from build123d import *

# Parameters (mm, degrees)
BOSS_EXTRUDE1_DEPTH       = 3.175
F_6_CLEARANCE_HOLE1_D     = 3.7973
F_6_CLEARANCE_HOLE1_DEPTH = 6.35
F_6_CLEARANCE_HOLE1_TIP   = 1.140824014
FILLET1_R                 = 1.27


with BuildPart() as part:
    # Sketch1 → Boss-Extrude1 (new body)
    with BuildSketch(Plane(origin=(0, 0, 0), x_dir=(1, 0, 0), z_dir=(0, 1, 0))):
        Polygon((-9.403419359, 20.244676918), (-9.403419359, 13.716876918), (-15.753419359, 13.716876918), (-15.753419359, 5.779376918), (-8.9789, 5.779376918), (-8.9789, 4.191876918), (14.904380641, 4.191876918), (14.904380641, 7.239876918), (8.376580641, 7.239876918), (8.376580641, 13.767676918), (14.904380641, 13.767676918), (14.904380641, 27.229676918), (8.376580641, 27.229676918), (8.376580641, 31.992176918), (-9.403419359, 31.992176918), (-9.403419359, 28.182176918), (-15.753419359, 28.182176918), (-15.753419359, 20.244676918), align=None)
        Polygon((-6.228419359, 8.001876918), (-6.228419359, 26.178617608), (3.752707316, 8.001876918), align=None, mode=Mode.SUBTRACT)
        Polygon((5.201580641, 28.817176918), (5.201580641, 10.640436229), (-4.779546034, 28.817176918), align=None, mode=Mode.SUBTRACT)
    extrude(amount=BOSS_EXTRUDE1_DEPTH)

    # 6 Clearance Hole1
    with Locations(Plane(origin=(11.855385862, 0, -6.482820987), x_dir=(-1, 0, 0), z_dir=(0, -1, 0))):
        with Locations((0.126005221, 16.809855931), (24.256005221, 18.145395592), (24.256005221, 3.857895592)):
            Hole(F_6_CLEARANCE_HOLE1_D / 2, depth=F_6_CLEARANCE_HOLE1_DEPTH)
            with Locations((0, 0, -(F_6_CLEARANCE_HOLE1_DEPTH + F_6_CLEARANCE_HOLE1_TIP / 2))):  # 118° drill point
                Cone(0, F_6_CLEARANCE_HOLE1_D / 2, F_6_CLEARANCE_HOLE1_TIP, mode=Mode.SUBTRACT)

    # Fillet1
    fillet1_edges = [part.edges().sort_by_distance(p)[0] for p in [
        (-6.228419359, 1.5875, -26.178617608),
        (-6.228419359, 1.5875, -8.001876918),
        (3.752707316, 1.5875, -8.001876918),
        (5.201580641, 1.5875, -10.640436229),
        (5.201580641, 1.5875, -28.817176918),
        (-4.779546034, 1.5875, -28.817176918),
    ]]
    fillet(fillet1_edges, radius=FILLET1_R)


solid = part.part
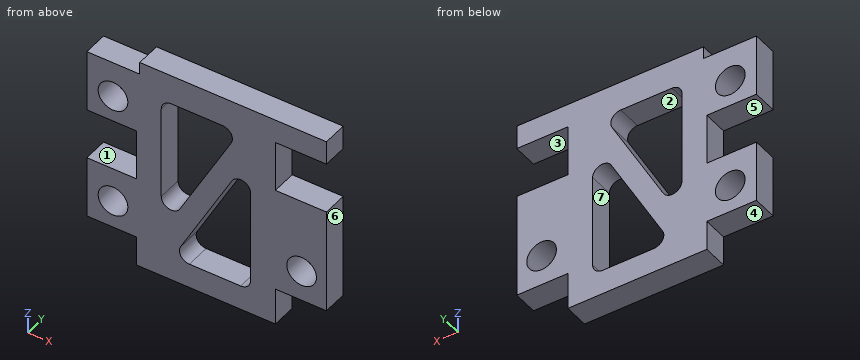
Geometry: final body of the model. Coordinates: model frame, mm. Face numbers are marked on the shaded views. A direction names the side the tool comes from. Round coordinates to 2 decimals unless told otherwise and drop trailing zeros. Order: outer loops, then holes, each group sorted by start corner. A loop starts at its lowest first (then second) coordinate and runs counter-clockwise, first axis right, second up.
Q1. Access query for the marked faces 1, 2, 3 and 4. Directions: +Z, -Z, +X, -X, +Y, -Y. A direction counts if a zero-diameter tool reaches every point of the face in a straight line with its end or side. Return the directions, or none.
Result sheet:
face 1: -X, +Y, -Y
face 2: +Y, -Y
face 3: +X, +Y, -Y
face 4: -Z, -X, +Y, -Y
Q2. Mould query, pull axis X, two halves, no side actions, for the marked faces 5, 6 and 7. Classes: released by +X, released by -X, zero draft, split by the parting line, or undercut.
Result sheet:
face 5: zero draft
face 6: released by +X
face 7: undercut
Q3. Section B-B, the plane y = 0.45. Give the number of separate pieces and of enclosed holes in the cut face, and give its area (3 significant figures).
Result sheet:
separate pieces: 1
enclosed holes: 5
area: 498 mm2
Q4. Pin query (flat end, axial travel): pin 1 (5 mm diameter, centred on x = -12.4, z = -10.34, fed in from +Y) (3 decimals); pin 2 (1 mm diameter, centred on x = 10.5, y = 1, fed in from -Z); pin 3 (1.6 mm diameter, centred on x = -11.5, y = 1.5, fed in from -Z); pin 4 (1.6 mm diameter, centred on y = 1.5, z = -12, fed in from +X). Return the tip coordinate at first contact, or that it passes through.
Result sheet:
pin 1: stops at y = 3.175
pin 2: stops at z = -27.23
pin 3: stops at z = -28.18
pin 4: stops at x = 8.38
Q5. Material intervals for probe 1 along Z at (x, y) = (9.5, 0.6); probe 2 along Z at (x, y) = (10.5, 2.3); probe 3 along X at (y, z) = (1.2, -23), sorted ascending.
Result sheet:
probe 1: z = -27.23 to -13.77, -7.24 to -4.19
probe 2: z = -27.23 to -24.74, -21.85 to -13.77, -7.24 to -4.19
probe 3: x = -15.75 to -13.38, -11.42 to -1.59, 5.2 to 9.85, 13.61 to 14.9
Q6. Section A-A, the plane x = 10.5. Output: boundary loops of the cut face in (y, z) (3 decimals), and give its area (3 significant figures).
Result sheet:
outline: (0, -27.23) - (3.175, -27.23) - (3.175, -24.74) - (0, -24.74) - close; (0, -21.846) - (3.175, -21.846) - (3.175, -13.768) - (0, -13.768) - close; (0, -7.24) - (3.175, -7.24) - (3.175, -4.192) - (0, -4.192) - close
area: 43.2 mm2
Q7. Section C-C, the plane z = -19.75. Output: boundary loops of the cut face in (x, y) (3 decimals), and give its area (3 significant figures).
Result sheet:
outline: (-9.403, 0) - (-6.228, 0) - (-6.228, 3.175) - (-9.403, 3.175) - close; (-2.698, 0) - (0.199, 0) - (0.199, 3.175) - (-2.698, 3.175) - close; (5.202, 0) - (14.904, 0) - (14.904, 3.175) - (5.202, 3.175) - close
area: 50.1 mm2
